Autodesk Inventor part; units mm, degrees
ref_plane "YZ Plane" through (0, 0, 0) normal (1, 0, 0) x (0, 1, 0)
ref_plane "XZ Plane" through (0, 0, 0) normal (0, 1, 0) x (-1, 0, 0)
ref_plane "XY Plane" through (0, 0, 0) normal (0, 0, 1) x (1, 0, 0)
sketch "Sketch1" plane through (0, 0, 0) normal (0, 0, 1) x (1, 0, 0)
  line L0 (14, 4) -> (14, 17.75)
  line L1 (14, 17.75) -> (18, 17.75) construction
  line L2 (18, 17.75) -> (18, 0)
  line L3 (3, 4) -> (3, 9)
  line L4 (3, 9) -> (0, 10)
  line L5 (3, 4) -> (14, 4)
  line L6 (14, 31.5) -> (14, 17.75)
  line L7 (18, 17.75) -> (18, 35.5)
  line L8 (3, 31.5) -> (3, 26.5)
  line L9 (3, 26.5) -> (0, 25.5)
  line L10 (3, 31.5) -> (14, 31.5)
  line L11 (-3.6, 0) -> (21.6, 0) construction
  line L12 (0, 35.5) -> (18, 35.5)
  line L13 (18, 0) -> (0, 0)
  line L14 (0, 35.5) -> (0, 25.5)
  line L15 (0, 0) -> (0, 10)
  dimension "d1" = 4
  dimension "d5" = 5
  dimension "d8" = 13.75
  dimension "d9" = 11
  dimension "d26" = 6
  dimension "d27" = 4
  dimension "d28" = 3
extrude "Extrusion1" add sketch "Sketch1" along normal blind 10
sketch "Sketch2" plane through (0, 0, 0) normal (0, 0, 1) x (1, 0, 0)
  circle A0 centre (23, 17.75) radius 5 construction
  line L0 (23, 17.75) -> (18, 17.75) construction
  arc A1 (18.6314, -3.2) -> (22.1621, 35.5) centre (10.6764, 17.0368) ccw
  arc A2 (18, 0) -> (20.4718, 32.7828) centre (10.6764, 17.0368) ccw
  arc A3 (18, 1.3146) -> (19.8379, 31.7639) centre (10.6764, 17.0368) ccw
  arc A4 (22.1621, 35.5) -> (19.8379, 31.7639) centre (21, 33.632) ccw
  arc A5 (21.5282, 34.4811) -> (20.4718, 32.7828) centre (21, 33.632) ccw
  line L1 (0, 0) -> (18, 0)
  line L2 (0, 2.0656) -> (0, 0)
  line L3 (18, 0) -> (18, 35.5)
  line L4 (18, 1.3146) -> (18, 0)
  line L5 (18, 0) -> (18, 35.5)
  arc A6 (18.4007, -2) -> (21.5282, 34.4811) centre (10.6764, 17.0368) ccw
  line L6 (0, 0) -> (18, 0)
  line L7 (18.4007, -2) -> (4, -2)
  line L8 (4, -2) -> (4, 0)
  line L9 (18.6314, -3.2) -> (0, -3.2)
  line L10 (0, -3.2) -> (0, 0)
  line L11 (29.1528, 15.4528) -> (31.1455, 15.282) construction
  dimension "d12" = 10
  dimension "d24" = 2.2
  dimension "d33" = 3
  dimension "d39" = 1.2
  dimension "d40" = 4
  dimension "d41" = 2
  dimension "d42" = 2
  dimension "d43" = 1.2
extrude "Extrusion2" add sketch "Sketch2" along normal blind 10 contours L9 L10 L1 L8 L7 A6 A5 A2 L3 A3 A4 A1
fillet "Fillet3" radius 1 5 edges at (18, 1.3146, 5) (18.4007, -2, 5) (4, 0, 5) (4, -2, 5) (18.6314, -3.2, 5)
fillet "Fillet4" radius 1 1 edges at (18, 35.5, 5)
properties part number "Clip"
Model file for the job. Use its own axes, mm. A direction names the side the tool comes from. Give positions to 0.01 mm unless a question says otherwise; leave off trailing zeros. Loops run counter-clockwise (first coordinate to the right, second up) from the corner with the lowest first, then second, coordinate; pieces in that order, holes last.
Item 1: Slice it at C-C (x = 7.5). Write the cut outline in (y, z).
Check values:
outline: (-3.2, 0) - (-2, 0) - (-2, 10) - (-3.2, 10) - close; (0, 0) - (4, 0) - (4, 10) - (0, 10) - close; (31.5, 0) - (35.5, 0) - (35.5, 10) - (31.5, 10) - close
Item 2: Drill centre lines: line 1 along Y through (x, z) = (11.5, 5); line 2 along X through (y, z) = (16.5, 4.5); line 3 along Y through (x, z) = (3.5, 7.75). Where is each one in solid material? Low to high.
Check values:
line 1: y = -3.2 to -2, 0 to 4, 31.5 to 35.5
line 2: x = 14 to 18, 28.01 to 29.21, 31.21 to 32.41
line 3: y = -3.2 to 4, 31.5 to 35.5
Item 3: Slice it at A-A (x = 16.5). Write the cut outline in (y, z).
Check values:
outline: (-3.2, 0) - (-2, 0) - (-2, 10) - (-3.2, 10) - close; (0, 0) - (35.5, 0) - (35.5, 10) - (0, 10) - close
Item 4: Drop flat-ended pins along their axis: P1, Ø5.5, axis at y = 7, z = 6, coming from the +X side; P2, Ø3, axis at y = 22.5, z = 4, coming from the -X side; P3, Ø5.5, axis at y = 29.5, z = 4.5, coming from the +X side. Give the stop position or say it passes through.
Check values:
P1: stops at x = 31.16
P2: stops at x = 14
P3: stops at x = 30.13
Item 5: Slice it at B-B (y = 18). Write the cut outline in (x, z), plus the area to 3 significant figures.
Check values:
outline: (14, 0) - (18, 0) - (18, 10) - (14, 10) - close; (27.99, 0) - (29.2, 0) - (29.2, 10) - (27.99, 10) - close; (31.2, 0) - (32.4, 0) - (32.4, 10) - (31.2, 10) - close
area: 64.0 mm2
Item 6: Which spindle directions (+Z, -Z, +X, -X, +Y, -Y) get a long thin tool onto all of the face, cutting with end or side? Do faces 4 (the face through (31.177, 15.697, 4.93)), 5 (the face through (17.715, 35.199, 5.07)), 6 (the face through (15, 15, 10)). Say none if no direction does.
Check values:
face 4: +Z, -Z
face 5: +Z, -Z, +Y
face 6: +Z, +X, -X, +Y, -Y
Item 7: Slice it at D-D (x = 24). Write the cut outline in (y, z).
Check values:
outline: (-0.15, 0) - (1.4, 0) - (1.4, 10) - (-0.15, 10) - close; (4.14, 0) - (5.93, 0) - (5.93, 10) - (4.14, 10) - close; (28.14, 0) - (29.94, 0) - (29.94, 10) - (28.14, 10) - close; (32.67, 0) - (34.22, 0) - (34.22, 10) - (32.67, 10) - close
Item 8: Mould opens along X. For faces 1 (the face through (8, 35.5, 5)), 2 (the face through (20.14, 34.14, 4.93)), 3 (the face through (0, 31, 5)) say: +X half, -X half, draft (parallel to the pull), parting line (faces both ways), or undercut.
Check values:
face 1: draft
face 2: undercut
face 3: -X half
